Here's how the part is built. I have some questions about the finished solid (model axes, mm). Face numbers are marked on the shaded views. A direction names the side the tool comes from. Round coordinates to 2 decimals unless told otherwise and drop trailing zeros. Order: outer loops, then holes, each group sorted by start corner. A loop starts at its lowest first (then second) coordinate and runs counter-clockwise, first axis right, second up. Notation, with made-up numbers: (-28, 52) - (-13, 52) arc R19 cw to (-13, 75) - close; hole circle Ø7 at (-37, 10). An arc over 180 degrees is marked (long way). Answer as a JSON object with one key per item and string values.
```python
from build123d import *

# Parameters (mm, degrees)
AUFSATZ_LINEAR_AUSTRAGEN1_DEPTH = 15
SKIZZE2_W                       = 14.1
SKIZZE2_H                       = 5
AUFSATZ_LINEAR_AUSTRAGEN2_DEPTH = 15
SKIZZE3_W                       = 14.1
SKIZZE3_H                       = 15.2
AUFSATZ_LINEAR_AUSTRAGEN3_DEPTH = 15


with BuildPart() as part:
    # Skizze1 → Aufsatz-Linear austragen1 (new body)
    with BuildSketch(Plane(origin=(0, 0, 0), x_dir=(1, 0, 0), z_dir=(0, 1, 0))):
        Polygon((-2, 12.1), (-2, -2), (54.1, -2), (54.1, 12.1), (33.1, 12.1), (33.1, 54.3), (19, 54.3), (19, 12.1), align=None)
        Polygon((0, 0), (52.1, 0), (52.1, 10.1), (31.1, 10.1), (31.1, 52.3), (21, 52.3), (21, 10.1), (0, 10.1), align=None, mode=Mode.SUBTRACT)
    extrude(amount=AUFSATZ_LINEAR_AUSTRAGEN1_DEPTH)

    # Skizze2 → Aufsatz-Linear austragen2 (add)
    with BuildSketch(Plane(origin=(0, 15, 0), x_dir=(1, 0, 0), z_dir=(0, 1, 0))):
        with Locations((26.05, 51.8)):
            Rectangle(SKIZZE2_W, SKIZZE2_H)
    extrude(amount=AUFSATZ_LINEAR_AUSTRAGEN2_DEPTH)

    # Skizze3 → Aufsatz-Linear austragen3 (add)
    with BuildSketch(Plane.XZ):
        with Locations((26.05, -46.7)):
            Rectangle(SKIZZE3_W, SKIZZE3_H)
    extrude(amount=-AUFSATZ_LINEAR_AUSTRAGEN3_DEPTH)


solid = part.part
```
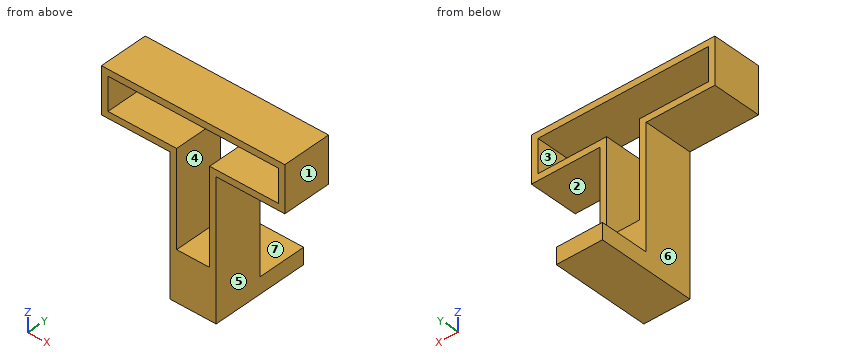
1. Imagine slicing it at D-D (x = 26.5). List the corners of the cut face in (y, z) for me, plus the area to 3 significant figures.
Responses:
{"outline": "(0, -54.3) - (30, -54.3) - (30, -49.3) - (15, -49.3) - (15, -39.1) - (0, -39.1) - close; (0, 0) - (15, 0) - (15, 2) - (0, 2) - close", "area": "333 mm2"}
2. Thinking about a two-plate mould opening in X: for the marked faces 1, 2 and 3, which applies, pulls with the +X half, pulls with the -X half, needs draft (parallel to the pull), parting line crosses it, or undercut?
Responses:
{"face 1": "pulls with the +X half", "face 2": "needs draft", "face 3": "undercut"}
3. Imagine slicing it at B-B (z = -4.5). List the corners of the cut face in (x, y) for me, plus the area to 3 significant figures.
Responses:
{"outline": "(-2, 0) - (0, 0) - (0, 15) - (-2, 15) - close; (52.1, 0) - (54.1, 0) - (54.1, 15) - (52.1, 15) - close", "area": "60.0 mm2"}
4. If I drill on L1, parallel to Z at x = 17.5, y = 8.75; L2, parallel to X at y = 4, z = -18; L3, parallel to X at y = 14, z = -11, over which ranges is the centre line in solid material (lowest first)? Write a range as [from, to].
Responses:
{"L1": "[-12.1, -10.1], [0, 2]", "L2": "[19, 21], [31.1, 33.1]", "L3": "[-2, 21], [31.1, 54.1]"}
5. Imagine slicing it at A-A (x = 50). List the corners of the cut face in (y, z) for me.
Responses:
{"outline": "(0, -12.1) - (15, -12.1) - (15, -10.1) - (0, -10.1) - close; (0, 0) - (15, 0) - (15, 2) - (0, 2) - close"}
6. Imagine slicing it at C-C (y = 9.5). List the corners of the cut face in (x, z) for me.
Responses:
{"outline": "(-2, -12.1) - (19, -12.1) - (19, -54.3) - (33.1, -54.3) - (33.1, -12.1) - (54.1, -12.1) - (54.1, 2) - (-2, 2) - close; hole (0, -10.1) - (21, -10.1) - (21, -39.1) - (31.1, -39.1) - (31.1, -10.1) - (52.1, -10.1) - (52.1, 0) - (0, 0) - close"}
7. For the marked faces 4, 5, 6 and 7, which set-ups out of +Z, -Z, +X, -X, +Y, -Y let a thin tool reach every point of the face, with its end or its side?
Responses:
{"face 4": "+Y, -Y", "face 5": "-Z, +X, +Y, -Y", "face 6": "-Z, -X, +Y, -Y", "face 7": "+Z, +X, -X, +Y"}
8. For P1, Ø16.5, axis at y = 9, z = -30, coming from the -X side; P2, Ø3, axis at x = 40.5, y = 12.5, coming from the -Z side; P3, Ø8, axis at x = 14.5, z = -34, coming from the +Y side; P4, Ø16.5, axis at y = 8, z = -30.5, coming from the +X side, each with a flat end and sliding along its axis, tell me the tip position at first contact or that it passes through.
Responses:
{"P1": "x = 19", "P2": "z = -12.1", "P3": "through", "P4": "x = 33.1"}
